Answer from the drawing. Dimensions are ordinates in mm from the lowest x, y and z of the part. A direction names the side the tool comes from. Coordinates: 2 decimals unless noted, no trailing zeros. Write each loop counter-clockwise with the first axis right and the second up, starting at its lowest first coordinate (ties: lowest second). Pieces come first, ordered by that corner, then holes. Notation, with made-up numbers: (75.5, 4.5) - (110.5, 4.5) arc R20 ccw to (110.5, 37.5) - close; hole circle Ø7 at (73.25, 58.25). An arc over 180 degrees is marked (long way). Use CSV: the item, a comma, the result in double quotes. Start each with the question number.
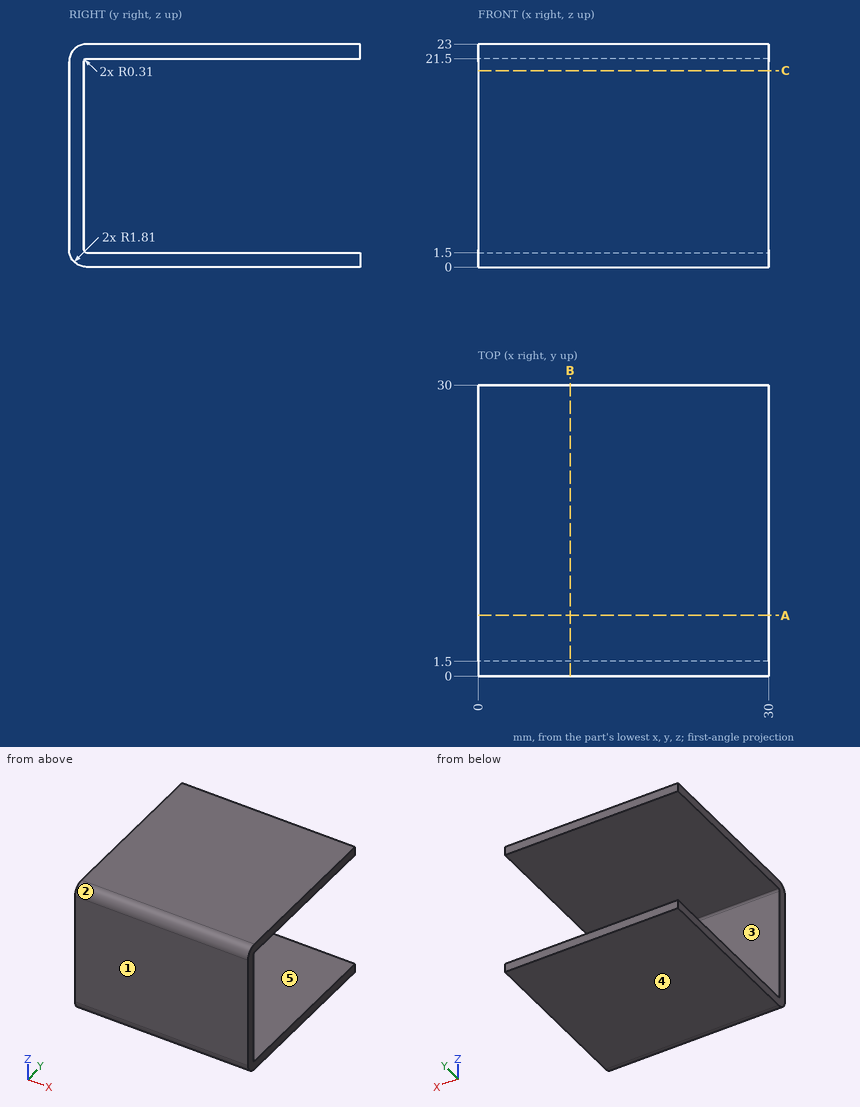
Item 1: Straight lines are drawn through the part: probe 1 along Z at (x, y) = (4.5, 12.5); probe 2 along Y at (x, z) = (21.75, 4.5); probe 3 along Y at (x, z) = (6.75, 22). For each, find the intervals that lie inside material, in ascending order. Write a range as [from, to].
Item 2: Which of the six approach directions +Z, -Z, +X, -X, +Y, -Y give full straight-line access (tool end or side, diameter ignored) to the marked faces 4 and 5?
Item 3: A cutting plane is placed at B-B (x = 9.5). Determine the outline of the cut face in (y, z), then the cut area to 3 significant figures.
Item 4: A cutting plane is placed at A-A (y = 6.25). Determine the outline of the cut face in (x, z), then the cut area to 3 significant figures.
Item 5: Determine the mould class of the marked faces 1, 2 and 3 for opening direction Z: +Z half, -Z half, draft (parallel to the pull), parting line (faces both ways), or undercut.
Item 6: A cutting plane is placed at C-C (z = 20.25). Determine the outline of the cut face in (x, y), then the cut area to 3 significant figures.
Item 7: This flat-tipped pin is pushed along its axis until it touches: pin 1 (6 mm diameter, centred on x = 16.5, z = 15, fed in from +Y). Where does it stop, or does it pass through?
Calculated:
1,probe 1,"z = [0, 1.5], [21.5, 23]"
1,probe 2,"y = [0, 1.5]"
1,probe 3,"y = [0.19, 30]"
2,face 4,"-Z, +X, -X, +Y, -Y"
2,face 5,"+X, -X, +Y"
3,outline,"(0, 1.81) arc R1.81 ccw to (1.81, 0) - (30, 0) - (30, 1.5) - (1.81, 1.5) arc R0.31 cw to (1.5, 1.81) - (1.5, 21.19) arc R0.31 cw to (1.81, 21.5) - (30, 21.5) - (30, 23) - (1.81, 23) arc R1.81 ccw to (0, 21.19) - close"
3,area,"119 mm²"
4,outline,"(0, 0) - (30, 0) - (30, 1.5) - (0, 1.5) - close; (0, 21.5) - (30, 21.5) - (30, 23) - (0, 23) - close"
4,area,"90.0 mm²"
5,face 1,"draft"
5,face 2,"+Z half"
5,face 3,"undercut"
6,outline,"(0, 0) - (30, 0) - (30, 1.5) - (0, 1.5) - close"
6,area,"45.0 mm²"
7,pin 1,"stops at y = 1.5"
